The model under review builds one solid part; all positions refer to its coordinate system, in mm. A direction names the side the tool comes from. Coordinates: 2 decimals unless noted, no trailing zeros. Write each loop counter-clockwise with the first axis right and the second up, starting at its lowest first coordinate (ties: lowest second). Pieces come first, ordered by that corner, then holes. Notation, with made-up numbers: (31, 38) - (89, 38) arc R21 ccw to (89, 62) - close; hole circle Ø1 at (-37, 48.5). An arc over 180 degrees is marked (long way). Return JSON: item names as keys, results as strings. Group by question number.
(1) Draft analysis for pull direction Z (two halves, no side actions). For faces 3 (the face through (-0.325, 3.721, 1.536)), 4 (the face through (6.2, 0.4, 0)), 5 (the face through (-0.325, -3.784, 1.536)), 6 (the face through (2.745, -0.022, 1.366)), state which applies: released by +Z, released by -Z, zero draft, split by the parting line, or undercut.
(2) We need section B-B on x = 0. State the section outline as (y, z) points.
(3) For pin 1 Ø2 at (x, z) = (-1, 2.5) entering from -Y; pin 2 Ø5 at (x, y) = (14, -16) entering from +Z; pin 3 Ø3 at (y, z) = (11.5, -2.5) entering from +X; pin 4 Ø2.5 at (x, y) = (-1, -0.5) entering from +Z, all flat-tipped, find the tip position at first contact; note any pin that passes through.
(4) We need section C-C on y = 0. State the section outline as (x, z) points, then the cut area to 3 significant figures.
(5) To check wall thickness, follow L1, parallel to Z at x = 0, y = 3.25; L2, parallel to Z at x = -17.5, y = -5.5; L3, parallel to X at y = 4, z = 1.75. State the ranges of each line that lie inside material, in increasing order. Write a range as from..to.
(6) Tool access review of faces 1 (the face through (0, 1.5, 1)), 2 (the face through (0, 0, -4)): name each direction out of +Z, -Z, +X, -X, +Y, -Y from which nothing blocks a thin tool from reaching the whole face with its end or side.
(7) We need section A-A on z = 0.75. State the section outline as (x, y) points, then the cut area to 3 significant figures.
```python
from build123d import *

# Parameters (mm, degrees)
F0_R     = 30
F0_R_2   = 6
F1_DEPTH = 4
F2_DEPTH = 6
F3_R     = 1.5
F4_DEPTH = 12.5
F5_W     = 4.6
F5_H     = 3
F6_DEPTH = 9.4


with BuildPart() as f1:
    # F0 (on Top) → F1 (new body)
    with BuildSketch(Plane.XY):
        Circle(F0_R)
        Circle(F0_R_2, mode=Mode.SUBTRACT)
        Circle(F0_R_2)
    extrude(amount=-F1_DEPTH)

    # F0 (on Top) → F2 (join)
    with BuildSketch(Plane.XY):
        Circle(F0_R_2)
    extrude(amount=F2_DEPTH)

    # F3 (on Front) → F4 (cut, symmetric)
    with BuildSketch(Plane.XZ):
        with Locations((0, 3)):
            Circle(F3_R)
    extrude(amount=F4_DEPTH, both=True, mode=Mode.SUBTRACT)

    # F5 (on face) → F6 (cut)
    with BuildSketch(Plane.XY.offset(6)):
        Rectangle(F5_W, F5_H)
        with BuildLine():
            ThreePointArc((-2.3, 1.5), (-2.7459060435, 0), (-2.3, -1.5))
            Line((-2.3, -1.5), (-2.3, 1.5))
        make_face()
        with BuildLine():
            Line((2.3, 1.5), (2.3, -1.5))
            ThreePointArc((2.3, -1.5), (2.745183651, 0), (2.3, 1.5))
        make_face()
    extrude(amount=-F6_DEPTH, mode=Mode.SUBTRACT)

    # F7 (on Front) → F8 (revolve, cut)
    with BuildSketch(Plane.XZ):
        Polygon((30, -3.4142135624), (30, -0.5857864376), (28.5857864376, -2), align=None)
    revolve(axis=Axis((0, 0, 0.7614716887), (0, 0, -1)), mode=Mode.SUBTRACT)


solid = f1.part
```
Ans:
{
 "1": {"face 3": "undercut", "face 4": "released by +Z", "face 5": "undercut", "face 6": "zero draft"},
 "2": {"outline": "(-30, -4) - (30, -4) - (30, -3.41) - (28.59, -2) - (30, -0.59) - (30, 0) - (6, 0) - (6, 1.5) - (1.5, 1.5) - (1.5, -3.4) - (-1.5, -3.4) - (-1.5, 1.5) - (-6, 1.5) - (-6, 0) - (-30, 0) - (-30, -0.59) - (-28.59, -2) - (-30, -3.41) - close; (-6, 4.5) - (-1.5, 4.5) - (-1.5, 6) - (-6, 6) - close; (1.5, 4.5) - (6, 4.5) - (6, 6) - (1.5, 6) - close"},
 "3": {"pin 1": "y = -5.97", "pin 2": "z = 0", "pin 3": "x = 28.17", "pin 4": "z = 6"},
 "4": {"outline": "(-30, -4) - (30, -4) - (30, -3.41) - (28.59, -2) - (30, -0.59) - (30, 0) - (6, 0) - (6, 6) - (2.75, 6) - (2.75, -3.4) - (-2.75, -3.4) - (-2.75, 6) - (-6, 6) - (-6, 0) - (-30, 0) - (-30, -0.59) - (-28.59, -2) - (-30, -3.41) - close", "area": "256 mm²"},
 "5": {"L1": "-4..1.5, 4.5..6", "L2": "-4..0", "L3": "-4.47..-0.83, 0.83..4.47"},
 "6": {"face 1": "+Z", "face 2": "-Z, +X, -X, +Y, -Y"},
 "7": {"outline": "circle Ø12 at (0, 0); hole (-2.3, -1.5) - (2.3, -1.5) arc R2.75 ccw to (2.3, 1.5) - (-2.3, 1.5) arc R2.75 ccw to start", "area": "97.5 mm²"}
}
